Here's the drawing with two shaded views (mm, measured from the low corner). I have some questions. Round coordinates to 2 decimals unless told otherwise and drop trailing zeros. Loops run counter-clockwise (first coordinate to the right, second up) from the corner with the lowest first, then second, coordinate; pieces in that order, holes last.
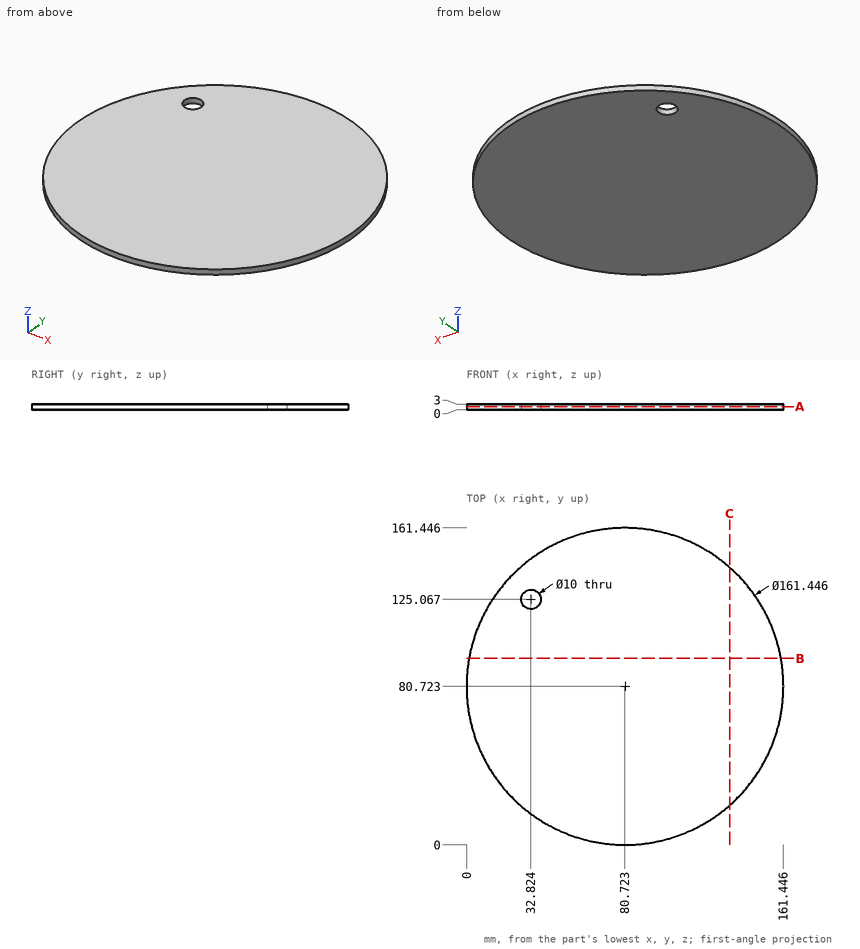
Item 1: If we section it at A-A, the plane z = 1.7: Please give me the cut outline in (x, y), then the cut area to 3 significant figures.
Results list:
outline: circle Ø161.45 at (80.72, 80.72); hole circle Ø10 at (32.82, 125.07)
area: 20,400 mm2
Item 2: If I drill on line 1 along Y through (x, z) = (85, 2.05); line 2 along X through (y, z) = (11, 0.7) (1 decimal); line 3 along X through (y, z) = (124, 0.1) (1 decimal), over which ranges is the centre line in solid material (lowest first)?
Results list:
line 1: y = 0.11 to 161.33
line 2: x = 40 to 121.4
line 3: x = 12.6 to 27.9, 37.7 to 148.9
Item 3: Will these pins go through, and if not, where does the flat tip stop? pin 1 (1 mm diameter, centred on y = 36.5, z = 1.5, fed in from -X); pin 2 (1 mm diameter, centred on x = 144, z = 1, fed in from +Y); pin 3 (1 mm diameter, centred on x = 114.5, z = 1.5, fed in from +Y); pin 4 (9 mm diameter, centred on x = 32.82, y = 125.07, fed in from -Z).
Results list:
pin 1: stops at x = 12.87
pin 2: stops at y = 131.47
pin 3: stops at y = 154.27
pin 4: passes through
Item 4: If we section it at C-C, the plane x = 134: Please give me the cut outline in (y, z).
Results list:
outline: (20.08, 0) - (141.37, 0) - (141.37, 3) - (20.08, 3) - close
Item 5: If we section it at B-B, the plane y = 95: Please give me the cut outline in (x, z), then the cut area to 3 significant figures.
Results list:
outline: (1.27, 0) - (160.17, 0) - (160.17, 3) - (1.27, 3) - close
area: 477 mm2
